Autodesk Inventor part; units mm, degrees
ref_plane "YZ Plane" through (0, 0, 0) normal (1, 0, 0) x (0, 1, 0)
ref_plane "XZ Plane" through (0, 0, 0) normal (0, 1, 0) x (-1, 0, 0)
ref_plane "XY Plane" through (0, 0, 0) normal (0, 0, 1) x (1, 0, 0)
sketch "Sketch1" plane through (0, 0, 0) normal (0, 1, 0) x (-1, 0, 0)
  line L0 (10, -35) -> (-10, -35)
  line L1 (-10, -35) -> (-10, 44.4211)
  line L2 (10, 44.4211) -> (10, -35)
  arc A0 (-10, 44.4211) -> (10, 44.4211) centre (0, 50.1) ccw
  point P0 (0, 0)
  dimension "d2" = 35
  dimension "d3" = 10
  dimension "d36" = 23
  dimension "d37" = 85.1
  dimension "d39" = 79.4211
  dimension "d40" = 20
extrude "Plate1" add sketch "Sketch1" along normal blind 1.5
sketch "Sketch3" plane through (0, 1.5, 0) normal (0, 1, 0) x (1, 0, 0)
  circle A0 centre (0, 25) radius 10
  circle A1 centre (0, -25) radius 10
  line L0 (-10, 35) -> (10, 35)
  line L1 (10, -44) -> (-10, -44)
  line L2 (-10, 35) -> (10, 35)
  line L3 (10, 35) -> (10, 25)
  line L4 (10, 25) -> (-10, 25)
  line L5 (-10, 25) -> (-10, 35)
  line L6 (10, -35) -> (-10, -35)
  line L7 (-10, -35) -> (-10, -25)
  line L8 (-10, -25) -> (10, -25)
  line L9 (10, -25) -> (10, -44)
  point P0 (0, 0)
  point P1 (-10, -44.4211)
  point P2 (10, -25)
  point P3 (0, -35)
  point P4 (-10, -35)
  point P5 (0, 35)
  point P6 (10, 35)
  dimension "d12" = 20
  dimension "d13" = 20
  dimension "d14" = 10
  dimension "d15" = 10
  dimension "d16" = 25
  dimension "d17" = 25
  dimension "d18" = 10
extrude "Extrusion1" cut sketch "Sketch3" against normal blind 10 contours L5 L0 A0 | A0 L0 L3
sketch "Sketch4" plane through (0, 1.5, 0) normal (0, 1, 0) x (1, 0, 0)
  circle A0 centre (-7, 25) radius 0.8
  arc A1 (10, 25) -> (-10, 25) centre (0, 25) ccw
  circle A2 centre (0, 18) radius 0.8
  circle A3 centre (7, 25) radius 0.8
  circle A4 centre (0, 32) radius 0.8
  point P0 (0, 0)
  dimension "d21" = 0
  dimension "d22" = 7
  dimension "d23" = 1.6
  dimension "d26" = 360
hole "Hole2" at (0, 1.5, -32) at (7, 1.5, -25) at (0, 1.5, -18) at (-7, 1.5, -25) direction (0, -1, 0) diameter 2.1 depth 1.5
fillet "Fillet1" radius 1 2 edges at (-10, 0.75, 44.4211) (10, 0.75, 44.4211)
sketch "Sketch5" plane through (0, 1.5, 0) normal (0, 1, 0) x (1, 0, 0)
  arc A0 (10, 25) -> (-10, 25) centre (0, 25) ccw
  point P0 (0, 0)
hole "Hole3" at (0, 1.5, -25) direction (0, -1, 0) diameter 7.2 depth 1.5
sketch "Sketch7" plane through (0, 1.5, 0) normal (0, 1, 0) x (1, 0, 0)
  circle A0 centre (7.525, -37.6) radius 1.05
  circle A1 centre (-7.525, -37.6) radius 1.05
  circle A2 centre (-7.525, -22.5) radius 1.05
  circle A3 centre (7.525, -22.5) radius 1.05
  point P0 (0, 0)
hole "Hole5" at (-7.525, 1.5, 22.5) at (7.525, 1.5, 22.5) at (7.525, 1.5, 37.6) at (-7.525, 1.5, 37.6) direction (0, -1, 0) diameter 2.1 end through all
equation "\"d33\" = Thickness"
equation "\"d47\" = Thickness"
equation "\"d61\" = Thickness"
equation "\"d4\" = Thickness"
equation "\"BendReliefWidth\" = Thickness"
equation "\"BendReliefDepth\" = 0.5 * Thickness"
equation "\"CornerReliefSize\" = 4 * Thickness"
equation "\"MinimumRemnant\" = 2 * Thickness"
equation "\"TransitionRadius\" = BendRadius"
equation "\"JacobiRadiusSize\" = BendRadius"
equation "\"GapSize\" = Thickness"
properties part number "axis_8_10_connector_frame" material "Aluminum 6061-AHC"
Could you check a few things on this model? Use its own coordinates, in mm. Give positions to 0.01 mm unless a question says otherwise; leave off trailing zeros. Write each loop counter-clockwise with the first axis right and the second up, starting at its lowest first coordinate (ties: lowest second). Pieces come first, ordered by that corner, then holes. Notation, with made-up numbers: (81.5, -0.5) - (125.5, -0.5) arc R22 ccw to (125.5, 22.5) - close; hole circle Ø9 at (59, 55). An arc over 180 degrees is marked (long way). Use CSV: the item, a comma, the result in double quotes. Start each with the question number.
Item 1: If we mould it in two halves opening along Z, with no side actions, what happens to faces 1 (the face through (0, 1.5, 4)), 2 (the face through (0.4, 0.74, -31.03)), 3 (the face through (-0.1, 0.7, 38.6))? For each: pulls with the +Z half, pulls with the -Z half, needs draft (parallel to the pull), parting line crosses it, or undercut.
Item 2: If I drill on line 1 along X through (y, z) = (0.65, 37.6) (3 decimals); line 2 along X through (y, z) = (0.65, -18); line 3 along Z through (x, y) = (7.5, 1.2), over which ranges is the centre line in solid material (lowest first)?
Item 3: I want a section at D-D, the plane y = 0.9. Give the number of separate pieces and of enclosed holes in the cut face, then the cut area to 3 significant figures.
Item 4: I want a section at A-A, the plane z = 37.6. Please give me the cut outline in (x, y) (3 decimals), then the cut area to 3 significant figures.
Item 5: I want a section at C-C, the plane x = 0. Please give me the cut outline in (y, z), then the cut area to 3 significant figures.
Item 6: I'm going to push flat-ended pins straight in: pin 1 (2.5 mm diameter, centred on x = -7.525, z = 22.5, fed in from +Y); pin 2 (6 mm diameter, centred on x = 0, z = -25, fed in from -Y). Where does each tip first touch, or does it pass through?
Item 7: I want a section at B-B, the plane z = -18. Please give me the cut outline in (x, y).
Findings:
1,face 1,"needs draft"
1,face 2,"undercut"
1,face 3,"pulls with the +Z half"
2,line 1,"x = -10 to -8.575, -6.475 to 6.475, 8.575 to 10"
2,line 2,"x = -10 to -1.05, 1.05 to 10"
2,line 3,"z = -31.61 to -25.92, -24.08 to 21.45, 23.55 to 36.55, 38.65 to 41.38"
3,separate pieces,"1"
3,enclosed holes,"9"
3,area,"1,390 mm2"
4,outline,"(-10, 0) - (-8.575, 0) - (-8.575, 1.5) - (-10, 1.5) - close; (-6.475, 0) - (6.475, 0) - (6.475, 1.5) - (-6.475, 1.5) - close; (8.575, 0) - (10, 0) - (10, 1.5) - (8.575, 1.5) - close"
4,area,"23.7 mm2"
5,outline,"(0, -35) - (1.5, -35) - (1.5, -33.05) - (0, -33.05) - close; (0, -30.95) - (1.5, -30.95) - (1.5, -28.6) - (0, -28.6) - close; (0, -21.4) - (1.5, -21.4) - (1.5, -19.05) - (0, -19.05) - close; (0, -16.95) - (1.5, -16.95) - (1.5, 38.6) - (0, 38.6) - close"
5,area,"93.3 mm2"
6,pin 1,"stops at y = 1.5"
6,pin 2,"passes through"
7,outline,"(-10, 0) - (-1.05, 0) - (-1.05, 1.5) - (-10, 1.5) - close; (1.05, 0) - (10, 0) - (10, 1.5) - (1.05, 1.5) - close"
